```python
from build123d import *

# Parameters (mm, degrees)
F0_W     = 27
F0_H     = 21
F0_R     = 1.75
F1_DEPTH = 5
F2_R     = 5
F3_R     = 1.75
F4_DEPTH = 1.5


with BuildPart() as f1:
    # F0 (on Top) → F1 (new body)
    with BuildSketch(Plane.XY):
        with Locations((8.77302, -3.012353)):
            Rectangle(F0_W, F0_H)
        with Locations((1.27302, -3.012353)):
            Circle(F0_R, mode=Mode.SUBTRACT)
        with Locations((16.27302, -3.012353)):
            Circle(F0_R, mode=Mode.SUBTRACT)
    extrude(amount=F1_DEPTH)

    # F2
    f2_edges = [f1.edges().sort_by_distance(p)[0] for p in [
        (-4.72698, -13.512353, 2.5),
        (22.27302, -13.512353, 2.5),
        (22.27302, 7.487647, 2.5),
        (-4.72698, 7.487647, 2.5),
    ]]
    fillet(f2_edges, radius=F2_R)

    # F3 (on face) → F4 (cut)
    with BuildSketch(Plane.XY.offset(5)):
        Polygon((4.27302, -4.744403), (4.27302, -1.280302), (1.27302, 0.451749), (-1.72698, -1.280302), (-1.72698, -4.744403), (1.27302, -6.476454), align=None)
        with Locations((1.27302, -3.012353)):
            Circle(F3_R, mode=Mode.SUBTRACT)
        Polygon((19.27302, -4.744403), (19.27302, -1.280302), (16.27302, 0.451749), (13.27302, -1.280302), (13.27302, -4.744403), (16.27302, -6.476454), align=None)
        with Locations((16.27302, -3.012353)):
            Circle(F3_R, mode=Mode.SUBTRACT)
    extrude(amount=-F4_DEPTH, mode=Mode.SUBTRACT)


solid = f1.part
```
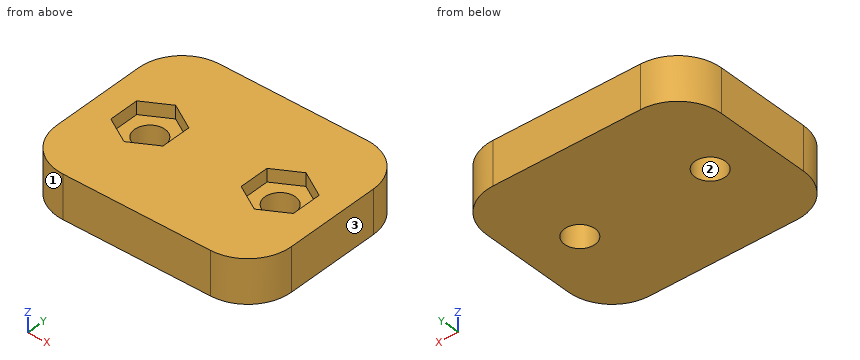
Geometry: final body of the model. Coordinates: model frame, mm. Face numbers are marked on the shaded views. Coordinates: 2 decimals unless noted, no trailing zeros. Order: outer loops, then holes, each group sorted by start corner. A loop starts at its lowest first (then second) coordinate and runs counter-clockwise, first axis right, second up. Notation, with made-up numbers: M 53.25,1 L 103.25,1 A37 ccw 103.25,38 Z; hole C 51,41 d10. An arc over 180 degrees is marked long. Answer in a Markdown table with one row per item. Add a question column.
Q1. Line query: L1, parallel to Y at x = 15, z = 3.55; L2, parallel to Y at x = 16, z = 3.8; L3, parallel to X at y = 2.75, z = 3.5. Output: solid intervals per line, ascending.
Q2. Section query D-D on z = 0.5. Return the cut outline in (x, y), and give its area (3 significant figures).
Q3. Contact query for a flat-ended pin moving along its axis: P1, Ø3, axis at x = 1.27, y = -3.01, coming from the -Z side. Output: stop coordinate, or through.
Q4. Section query C-C on x = -2.5. Return the cut outline in (y, z), and give its area (3 significant figures).
Q5. Section query A-A on z = 4.5. Return the cut outline in (x, y), and give its area (3 significant figures).
Q6. Section query B-B on y = -5.25. Return the cut outline in (x, z), and give its area (3 significant figures).
Q7. Mould query, pull axis X, two halves, no side actions, for the marked faces 1, 2 and 3. Classes: released by +X, released by -X, zero draft, split by the parting line, or undercut.
Completed:
| question | item | result |
|---|---|---|
| 1 | L1 | y = -13.51 to -5.74, -0.28 to 7.49 |
| 1 | L2 | y = -13.51 to -6.32, 0.29 to 7.49 |
| 1 | L3 | x = -4.72 to 22.27 |
| 2 | outline | M -4.73,-8.51 A5 ccw 0.27,-13.51 L 17.27,-13.51 A5 ccw 22.27,-8.51 L 22.27,2.49 A5 ccw 17.27,7.49 L 0.27,7.49 A5 ccw -4.73,2.49 Z; hole C 1.27,-3.01 d3.5; hole C 16.27,-3.01 d3.5 |
| 2 | area | 526 mm2 |
| 3 | P1 | passes through |
| 4 | outline | M -12.67,0 L 6.65,0 L 6.65,5 L -12.67,5 Z |
| 4 | area | 96.6 mm2 |
| 5 | outline | M -4.73,-8.51 A5 ccw 0.27,-13.51 L 17.27,-13.51 A5 ccw 22.27,-8.51 L 22.27,2.49 A5 ccw 17.27,7.49 L 0.27,7.49 A5 ccw -4.73,2.49 Z; hole M -1.73,-4.74 L 1.27,-6.48 L 4.27,-4.74 L 4.27,-1.28 L 1.27,0.45 L -1.73,-1.28 Z; hole M 13.27,-4.74 L 16.27,-6.48 L 19.27,-4.74 L 19.27,-1.28 L 16.27,0.45 L 13.27,-1.28 Z |
| 5 | area | 483 mm2 |
| 6 | outline | M -4.73,0 L 22.27,0 L 22.27,5 L 18.4,5 L 18.4,3.5 L 14.15,3.5 L 14.15,5 L 3.4,5 L 3.4,3.5 L -0.85,3.5 L -0.85,5 L -4.73,5 Z |
| 6 | area | 122 mm2 |
| 7 | face 1 | released by -X |
| 7 | face 2 | undercut |
| 7 | face 3 | released by +X |
